```python
from build123d import *

# Parameters (mm, degrees)
F0_R     = 2.159
F1_DEPTH = 3.175


with BuildPart() as f1:
    # F0 (on Front) → F1 (new body)
    with BuildSketch(Plane.XZ):
        with BuildLine():
            Line((-247.65, -25.4), (247.65, -25.4))
            ThreePointArc((247.65, -25.4), (252.140128, -23.540128), (254, -19.05))
            Line((254, -19.05), (254, 19.05))
            ThreePointArc((254, 19.05), (252.140128, 23.540128), (247.65, 25.4))
            Line((247.65, 25.4), (222.25, 25.4))
            Line((222.25, 25.4), (222.25, 6.35))
            Line((222.25, 6.35), (228.6, 6.35))
            ThreePointArc((228.6, 6.35), (234.95, 0), (228.6, -6.35))
            Line((228.6, -6.35), (215.9, -6.35))
            ThreePointArc((215.9, -6.35), (211.370438, -4.450345), (209.550988, 0.112025))
            Line((209.550988, 0.112025), (209.550988, 25.4))
            Line((209.550988, 25.4), (-209.550988, 25.4))
            Line((-209.550988, 25.4), (-209.550988, 0.112025))
            ThreePointArc((-209.550988, 0.112025), (-211.370438, -4.450345), (-215.9, -6.35))
            Line((-215.9, -6.35), (-228.6, -6.35))
            ThreePointArc((-228.6, -6.35), (-234.95, 0), (-228.6, 6.35))
            Line((-228.6, 6.35), (-222.25, 6.35))
            Line((-222.25, 6.35), (-222.25, 25.4))
            Line((-222.25, 25.4), (-247.65, 25.4))
            ThreePointArc((-247.65, 25.4), (-252.140128, 23.540128), (-254, 19.05))
            Line((-254, 19.05), (-254, -19.05))
            ThreePointArc((-254, -19.05), (-252.140128, -23.540128), (-247.65, -25.4))
        make_face()
        with Locations((-114.3, 0)):
            Circle(F0_R, mode=Mode.SUBTRACT)
        with Locations((114.3, 0)):
            Circle(F0_R, mode=Mode.SUBTRACT)
    extrude(amount=F1_DEPTH)


solid = f1.part
```
Build history of the part. All positions in model axes, mm. Give positions to 0.01 mm unless a question says otherwise; leave off trailing zeros. Order: outer loops, then holes, each group sorted by start corner. A loop starts at its lowest first (then second) coordinate and runs counter-clockwise, first axis right, second up. Notation, with made-up numbers: M -3,60 L 5,60 A16 cw 5,81 Z; hole C 60,-31 d5. An arc over 180 degrees is marked long. Write item = value, one per line. Start each with the question number.
(1) Pin check, flat tips, straight feed: pin 1 Ø1.6 at (x, y) = (221, -1) entering from +Z; pin 2 Ø2.5 at (x, z) = (-114.3, 0) entering from -Y. Stop position of each tip, or through.
(2) Probe L1, parallel to X at y = -2.2, z = 13; L2, parallel to Z at x = -114.3, y = -2.5; L3, parallel to Z at x = 226, y = -2.8. List the from-to ranges inside material, lowest first. Write a range as [from, to].
(3) Slice it at A-A on y = -1.95. Write the cut outline in (x, z).
Responses:
q1.pin_1 = -6.35
q1.pin_2 = through
q2.L1 = [-254, -222.25], [-209.55, 209.55], [222.25, 254]
q2.L2 = [-25.4, -2.16], [2.16, 25.4]
q2.L3 = [-25.4, -6.35], [6.35, 25.4]
q3.outline = M -254,-19.05 A6.35 ccw -247.65,-25.4 L 247.65,-25.4 A6.35 ccw 254,-19.05 L 254,19.05 A6.35 ccw 247.65,25.4 L 222.25,25.4 L 222.25,6.35 L 228.6,6.35 A6.35 cw 228.6,-6.35 L 215.9,-6.35 A6.35 cw 209.55,0.11 L 209.55,25.4 L -209.55,25.4 L -209.55,0.11 A6.35 cw -215.9,-6.35 L -228.6,-6.35 A6.35 cw -228.6,6.35 L -222.25,6.35 L -222.25,25.4 L -247.65,25.4 A6.35 ccw -254,19.05 Z; hole C -114.3,0 d4.32; hole C 114.3,0 d4.32
